Design review of the part built by this model. Coordinates are the model's own, in mm. Face numbers are marked on the shaded views. Coordinates: 2 decimals unless noted, no trailing zeros. Loops run counter-clockwise (first coordinate to the right, second up) from the corner with the lowest first, then second, coordinate; pieces in that order, holes last. Notation, with made-up numbers: (-6, 6) -> (19, 6) arc R18 ccw to (19, 16) -> close; hole circle Ø2 at (43.5, -18.75). An arc over 180 degrees is marked (long way). Use one line per item in the form item = value. Start each with the question number.
1. Consider section A-A (z = 0). State the section outline as (x, y) points.
2. For pin 1 (6 mm diameter, centred on x = 35.5, y = 40, fed in from +Z); pin 2 (6 mm diameter, centred on x = 109.5, z = -25.5, fed in from -Y); pin 3 (1.5 mm diameter, centred on y = -35.5, z = 68.5, fed in from +X), all flat-tipped, find the tip position at first contact; note any pin that passes through.
3. The part is to be moulded in two halves that separate along Z. For the marked faces 1 and 2, say which applies: released by +Z, released by -Z, zero draft, split by the parting line, or undercut.
4. Wall thickness on line 1 (Z direction, x = 91.5, y = 0); line 2 (Z direction, x = 28, y = 0); line 3 (Y direction, x = 113, z = -51.5): over which ranges is each line inside the solid? List them lowest first. Write a range as from..to.
5. Consider section C-C (x = 63). State the section outline as (y, z) points.
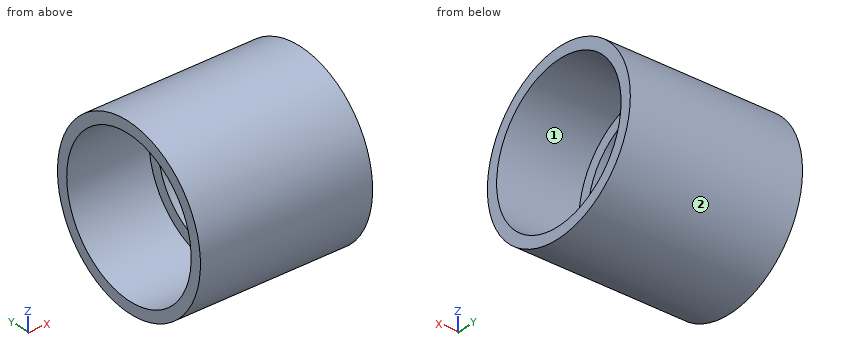
Autodesk Inventor part; units mm, degrees
ref_plane "YZ Plane" through (0, 0, 0) normal (1, 0, 0) x (0, 1, 0)
ref_plane "XZ Plane" through (0, 0, 0) normal (0, 1, 0) x (-1, 0, 0)
ref_plane "XY Plane" through (0, 0, 0) normal (0, 0, 1) x (1, 0, 0)
sketch "Sketch1" plane through (0, 0, 0) normal (0, 0, 1) x (1, 0, 0)
  line L0 (0, 0) -> (180, 0)
  line L1 (0, 0) -> (0, 80) construction
  line L2 (0, 80) -> (0, 91.9)
  line L3 (0, 91.9) -> (180, 91.9)
  line L4 (0, 80) -> (86, 80)
  line L5 (86, 80) -> (86, 68.1)
  line L6 (86, 68.1) -> (94, 68.1)
  line L7 (90, 0) -> (90, 91.9) construction
  line L8 (180, 0) -> (180, 80) construction
  line L9 (180, 80) -> (180, 91.9)
  line L10 (180, 80) -> (94, 80)
  line L11 (94, 80) -> (94, 68.1)
  line L12 (86, 68.1) -> (86, 0) construction
  line L13 (94, 68.1) -> (94, 0) construction
  dimension "d0" = 160
  dimension "d2" = 11.9
  dimension "d3" = 8
  dimension "d4" = 86
  dimension "d5" = 11.9
revolve "Revolution1" add sketch "Sketch1" angle 360 about axis through (0, 0, 0) along (1, 0, 0)
equation "\"d0\" = d1"
equation "\"d2\" = s1"
equation "\"d3\" = z1"
equation "\"d4\" = t1"
equation "\"d5\" = s1"
equation "\"d1\" = 160"
equation "\"t1\" = 86"
equation "\"z1\" = 8"
equation "\"s1\" = 11.9"
properties part number "DIN 8063 Муфта, тип M 160" material "ПВХ, непластифицированный"
Geometry check:
q1.outline = (0, -91.9) -> (180, -91.9) -> (180, -80) -> (94, -80) -> (94, -68.1) -> (86, -68.1) -> (86, -80) -> (0, -80) -> close; (0, 80) -> (86, 80) -> (86, 68.1) -> (94, 68.1) -> (94, 80) -> (180, 80) -> (180, 91.9) -> (0, 91.9) -> close
q2.pin_1 = 84.12
q2.pin_2 = -89.1
q2.pin_3 = 94
q3.face_1 = undercut
q3.face_2 = split by the parting line
q4.line_1 = -91.9..-68.1, 68.1..91.9
q4.line_2 = -91.9..-80, 80..91.9
q4.line_3 = -76.11..-61.22, 61.22..76.11
q5.outline = circle Ø183.8 at (0, 0); hole circle Ø160 at (0, 0)
